Check sheet for the modelled part. Datum: model origin and axes. Units: mm. A direction names the side the tool comes from. Coordinates: 2 decimals unless noted, no trailing zeros. Loops run counter-clockwise (first coordinate to the right, second up) from the corner with the lowest first, then second, coordinate; pieces in that order, holes last. Notation, with made-up numbers: (-20, 77.5) -> (-6, 77.5) arc R34 ccw to (-6, 110.5) -> close; hole circle Ø7 at (29.25, 48). An arc over 180 degrees is marked (long way). Use CSV: the item, a comma, the result in double quotes.
Autodesk Inventor part; units mm, degrees
ref_plane "YZ Plane" through (0, 0, 0) normal (1, 0, 0) x (0, 1, 0)
ref_plane "XZ Plane" through (0, 0, 0) normal (0, 1, 0) x (-1, 0, 0)
ref_plane "XY Plane" through (0, 0, 0) normal (0, 0, 1) x (1, 0, 0)
sketch "Sketch1" plane through (0, 0, 0) normal (0, 1, 0) x (-1, 0, 0)
  line L0 (0, 0) -> (100, 0)
  line L1 (100, 0) -> (100, -75)
  line L2 (100, -75) -> (0, -75)
  line L3 (0, -75) -> (0, 0)
  line L4 (100, -75) -> (100, 0)
  dimension "d0" = 100
  dimension "d1" = 75
extrude "Extrusion1" add sketch "Sketch1" along normal blind 12
sketch "Sketch2" plane through (0, 0, 0) normal (1, 0, 0) x (0, 0, -1)
  line L0 (0, 0) -> (75, 0)
  line L1 (30, 0) -> (45, 0)
  line L2 (45, 0) -> (45, 10)
  line L3 (45, 10) -> (30, 10)
  line L4 (30, 10) -> (30, 0)
  line L5 (75, 0) -> (75, 12)
  line L6 (0, 0) -> (0, 12)
  point P0 (0, 6)
  point P1 (30, 5)
  point P2 (45, 0)
  dimension "d12" = 15
  dimension "d13" = 75
  dimension "d14" = 30
  dimension "d15" = 10
extrude "Extrusion2" cut sketch "Sketch2" against normal through all
sketch "Sketch3" plane through (-100, 0, 0) normal (0, 0, 1) x (1, 0, 0)
  line L0 (0, 0) -> (0, 12)
  line L1 (15, 4) -> (75, 4) construction
  line L2 (15, 1.9) -> (75, 1.9)
  line L3 (75, 6.1) -> (15, 6.1)
  arc A0 (15, 6.1) -> (15, 1.9) centre (15, 4) ccw
  arc A1 (75, 1.9) -> (75, 6.1) centre (75, 4) ccw
  line L4 (0, 0) -> (100, 0)
  line L5 (0, 12) -> (100, 12)
  point P0 (0, 6)
  point P1 (45, 4)
  point P2 (0, 6)
  dimension "d20" = 4.2
  dimension "d21" = 15
  dimension "d22" = 4
  dimension "d23" = 12
  dimension "d60" = 60
extrude "Extrusion3" cut sketch "Sketch3" against normal through all
sketch "Sketch4" plane through (0, 0, -75) normal (1, 0, 0) x (0, 0, -1)
  circle A0 centre (-27.5, 9.5) radius 1.5
  line L0 (-30, 0) -> (0, 0)
  line L1 (-30, 10) -> (-30, 0)
  line L2 (-30, 0) -> (-45, 0) construction
  line L3 (-45, 0) -> (-37.5, 0) construction
  line L4 (-37.5, 0) -> (-37.5, -2.8944) construction
  circle A1 centre (-47.5, 9.5) radius 1.5
  line L5 (-75, 12) -> (0, 12)
  point P0 (-75, 0)
  dimension "d26" = 3
  dimension "d29" = 2.5
  dimension "d30" = 2.5
hole "Hole1" at (0, 9.5, -27.5) at (0, 9.5, -47.5) direction (-1, 0, 0) diameter 2.459 depth 8 tip angle 118
chamfer "Chamfer2" distance 0.4 angle 45 2 edges at (0, 9.5, -46.2705) (0, 9.5, -26.2705)
sketch "Sketch6" plane through (0, 12, 0) normal (0, 1, 0) x (1, 0, 0)
  circle A0 centre (-96, 21.66) radius 1
  line L0 (-100, 0) -> (0, 0)
  line L1 (-100, 75) -> (-100, 0)
  line L2 (-100, 37.5) -> (-44.6159, 37.5) construction
  line L3 (-50, 0) -> (-50, 87.3463) construction
  circle A1 centre (-4, 21.66) radius 1
  circle A2 centre (-96, 53.34) radius 1
  circle A3 centre (-4, 53.34) radius 1
  point P0 (-96, 21.66)
  point P1 (-4, 21.66)
  point P2 (-4, 21.66)
  point P3 (-96, 53.34)
  point P4 (-4, 53.34)
  point P5 (-4, 53.34)
  dimension "d49" = 2
  dimension "d50" = 21.66
  dimension "d52" = 4
hole "Hole3" at (-96, 12, -21.66) at (-96, 12, -53.34) at (-4, 12, -53.34) at (-4, 12, -21.66) direction (0, -1, 0) diameter 3.2 depth 13 tip angle 118 counterbore diameter 7.2 counterbore depth 4
sketch "Sketch8" plane through (0, 12, 0) normal (0, 1, 0) x (1, 0, 0)
  circle A0 centre (-95, 70) radius 2
  line L0 (0, 0) -> (0, 75) construction
  line L1 (0, 37.5) -> (-49.0535, 37.5) construction
  line L2 (-100, 75) -> (-100, 0)
  line L3 (0, 75) -> (-100, 75)
  line L4 (-66.5, 46.7026) -> (-66.5, 27.8899) construction
  circle A1 centre (-38, 70) radius 2
  point P0 (-38, 70)
  dimension "d61" = 4
  dimension "d75" = 5
  dimension "d76" = 57
  dimension "d77" = 5
hole "Hole4" at (-95, 12, -70) at (-38, 12, -70) direction (0, -1, 0) diameter 2.459 depth 8 tip angle 118
chamfer "Chamfer3" distance 0.4 angle 45 2 edges at (-95, 12, -71.2295) (-38, 12, -71.2295)
equation "\"d22\" = 0.333333 * d23"
equation "\"d29\" = d28"
properties part number "blat" material "Stainless Steel, Austenitic"
1) Go/stop test with flat-tipped pins: pin 1 Ø8 at (x, z) = (-31.5, -62.5) entering from -Y; pin 2 Ø4.5 at (x, z) = (-31, -38) entering from -Y; pin 3 Ø3 at (y, z) = (9.5, -47.5) entering from +X. Record where each tip stops, or that it passes through.
Answer below:
pin 1,"stops at y = 0"
pin 2,"stops at y = 10"
pin 3,"stops at x = -0.13"
2) Thickness scan on line 1 along Z through (x, y) = (-8, 9.75); line 2 along Z through (x, y) = (-96, 2.5); line 3 along X through (y, z) = (8.95, -53.34). Record the ranges inside material, lowest first. Write a range as from..to.
Answer below:
line 1,"z = -75..-48.7, -46.3..-45, -30..-28.7, -26.3..0"
line 2,"z = -75..-54.94, -51.74..-45, -30..-23.26, -20.06..0"
line 3,"x = -100..-99.6, -92.4..-7.6, -0.4..0"
3) Draft check along Y on faces 6 (the flat face through (-94, 8, -53)), 7 (the cylindrical face through (-4.07, 3.94, -54.94)), 8 (the cylindrical face through (-87.1, 4, -59.8)), 9 (the flat face through (-49, 10, -38)). Enter one of: released by +Y, released by -Y, zero draft, split by the parting line, or undercut.
Answer below:
face 6,"released by +Y"
face 7,"zero draft"
face 8,"undercut"
face 9,"released by -Y"
4) Access from +Z, -Z, +X, -X, +Y, -Y to the whole of each face (thin tool, end or side, straight path). Record for faces 1 (the flat face through (-55, 1.9, -60)), 2 (the flat face through (-2, 8, -53)), 3 (the flat face through (-49, 0, -15)), 4 (the cylindrical face through (-4.253, 9.971, -28.636)), 5 (the flat face through (-49, 7, -30)).
Answer below:
face 1,"+Z, -Z"
face 2,"+Y"
face 3,"+Z, -Z, +X, -X, -Y"
face 4,"+X"
face 5,"+X, -X, -Y"
5) Cross-section at B-B on z = -21.66. Record the boundary of the cut face in (x, y), and give its area (3 significant figures).
Answer below:
outline,"(-100, 0) -> (-97.6, 0) -> (-97.6, 8) -> (-99.6, 8) -> (-99.6, 12) -> (-100, 12) -> close; (-94.4, 0) -> (-5.6, 0) -> (-5.6, 8) -> (-7.6, 8) -> (-7.6, 12) -> (-92.4, 12) -> (-92.4, 8) -> (-94.4, 8) -> close; (-2.4, 0) -> (0, 0) -> (0, 12) -> (-0.4, 12) -> (-0.4, 8) -> (-2.4, 8) -> close; hole (-85, 1.9) -> (-25, 1.9) arc R2.1 ccw to (-25, 6.1) -> (-85, 6.1) arc R2.1 ccw to start"
area,"825 mm²"
6) Cross-section at C-C on x = -38. Record the boundary of the cut face in (y, z).
Answer below:
outline,"(0, -75) -> (1.9, -75) -> (1.9, -45) -> (0, -45) -> close; (0, -30) -> (1.9, -30) -> (1.9, 0) -> (0, 0) -> close; (6.1, -75) -> (12, -75) -> (12, -71.63) -> (11.6, -71.23) -> (6.1, -71.23) -> close; (6.1, -68.77) -> (11.6, -68.77) -> (12, -68.37) -> (12, 0) -> (6.1, 0) -> (6.1, -30) -> (10, -30) -> (10, -45) -> (6.1, -45) -> close"
7) Cross-section at A-A on x = -4. Record the boundary of the cut face in (y, z), and give its area (3 significant figures).
Answer below:
outline,"(0, -75) -> (12, -75) -> (12, -56.94) -> (8, -56.94) -> (8, -54.94) -> (0, -54.94) -> close; (0, -51.74) -> (8, -51.74) -> (8, -49.74) -> (12, -49.74) -> (12, -25.26) -> (8, -25.26) -> (8, -23.26) -> (0, -23.26) -> (0, -30) -> (10, -30) -> (10, -45) -> (0, -45) -> close; (0, -20.06) -> (8, -20.06) -> (8, -18.06) -> (12, -18.06) -> (12, 0) -> (0, 0) -> close; hole circle Ø2.46 at (9.5, -47.5); hole circle Ø2.46 at (9.5, -27.5)"
area,"632 mm²"
8) Cross-section at D-D on z = -11. Record the boundary of the cut face in (x, y).
Answer below:
outline,"(-100, 0) -> (0, 0) -> (0, 12) -> (-100, 12) -> close; hole (-85, 1.9) -> (-25, 1.9) arc R2.1 ccw to (-25, 6.1) -> (-85, 6.1) arc R2.1 ccw to start"
